Geometry: final body of the model. Coordinates: model frame, mm. Face numbers are marked on the shaded views. A direction names the side the tool comes from. Round coordinates to 2 decimals unless told otherwise and drop trailing zeros. Write each loop counter-clockwise with the first axis right and the second up, starting at its lowest first coordinate (ties: lowest second). Pieces come first, ordered by that corner, then holes. Notation, with made-up numbers: (48, -13) -> (77, -13) arc R15 ccw to (77, 9) -> close; hole circle Ø9 at (53, -15). An arc over 180 degrees is marked (long way). Use one line per item in the form item = value. Start each with the question number.
1. Pin query (flat end, axial travel): pin 1 Ø6 at (y, z) = (8, 1) entering from +X; pin 2 Ø2 at (x, z) = (10, -4) entering from +Y; pin 3 Ø1.6 at (x, y) = (-12, -111.5) entering from +Z. Return the tip coordinate at first contact, or that it passes through.
2. Cut plane B-B, the plane z = -2. Return the cut outline in (x, y).
3. Draft query along Y for the marked faces 3, 4 and 5. Return one class per face: pulls with the +Y half, pulls with the -Y half, needs draft (parallel to the pull), parting line crosses it, or undercut.
4. Cut plane C-C, the plane y = 5. Return the cut outline in (x, z), plus the area to 3 significant figures.
5. Line query: L1, parallel to X at y = -138.5, z = 2.75; L2, parallel to X at y = -138.5, z = 3.75; L3, parallel to Y at x = 7.5, z = -0.75. Output: solid intervals per line, ascending.
6. Reachability of the marked faces 1 and 2 from +Z, -Z, +X, -X, +Y, -Y: full face, straight path, thin tool, end or side. Return the list, or none.
```python
from build123d import *

# Parameters (mm, degrees)
F1_DEPTH = 150
F2_R     = 1.99999
F4_DEPTH = 12.2
F5_DEPTH = 25


# Not quite as in the source:
# - a fillet or chamfer is up to 0.001 mm smaller than in the source, because OpenCascade refuses the exact size


with BuildPart() as f1:
    # F0 (on Front) → F1 (new body)
    with BuildSketch(Plane.XZ):
        with BuildLine():
            ThreePointArc((20, 4.1), (19.4142135624, 5.5142135624), (18, 6.1))
            Line((18, 6.1), (16.25, 6.1))
            ThreePointArc((16.25, 6.1), (15.5428932188, 5.8071067812), (15.25, 5.1))
            Line((15.25, 5.1), (15.25, 3.1))
            Line((15.25, 3.1), (9.25, 3.1))
            Line((9.25, 3.1), (9.25, 5.1))
            ThreePointArc((9.25, 5.1), (8.9571067812, 5.8071067812), (8.25, 6.1))
            Line((8.25, 6.1), (-8.25, 6.1))
            ThreePointArc((-8.25, 6.1), (-8.9571067812, 5.8071067812), (-9.25, 5.1))
            Line((-9.25, 5.1), (-9.25, 3.1))
            Line((-9.25, 3.1), (-15.25, 3.1))
            Line((-15.25, 3.1), (-15.25, 5.1))
            ThreePointArc((-15.25, 5.1), (-15.5428932188, 5.8071067812), (-16.25, 6.1))
            Line((-16.25, 6.1), (-18, 6.1))
            ThreePointArc((-18, 6.1), (-19.4142135624, 5.5142135624), (-20, 4.1))
            Line((-20, 4.1), (-20, -4.1))
            ThreePointArc((-20, -4.1), (-19.4142135624, -5.5142135624), (-18, -6.1))
            Line((-18, -6.1), (18, -6.1))
            ThreePointArc((18, -6.1), (19.4142135624, -5.5142135624), (20, -4.1))
            Line((20, -4.1), (20, 4.1))
        make_face()
    extrude(amount=F1_DEPTH)

    # F2 (radius 2 in the source; OpenCascade refuses exactly that, so slightly less here)
    f2_edges = [f1.edges().sort_by_distance(p)[0] for p in [
        (15.25, -75, 3.1),
        (9.25, -75, 3.1),
        (-9.25, -75, 3.1),
        (-15.25, -75, 3.1),
    ]]
    fillet(f2_edges, radius=F2_R)

    # F3 (on face) → F4 (join)
    with BuildSketch(Plane(origin=(0, 0, -6.1), x_dir=(1, 0, 0), z_dir=(0, 0, -1))):
        with BuildLine():
            Line((0, 0), (-2.5, 0))
            Line((-2.5, 0), (-2.5, -6.5456439427))
            ThreePointArc((-2.5, -6.5456439427), (-1.2794263668, -6.1379979383), (0, -6))
            Line((0, -6), (0, 0))
        make_face()
        with BuildLine():
            Line((2.5, -6.5456439427), (2.5, 0))
            Line((2.5, 0), (0, 0))
            Line((0, 0), (0, -6))
            ThreePointArc((0, -6), (1.2794263668, -6.1379979383), (2.5, -6.5456439427))
        make_face()
        with BuildLine():
            Line((2.5, -8.2583426132), (2.5, -6.5456439427))
            ThreePointArc((2.5, -6.5456439427), (1.2794263668, -6.1379979383), (0, -6))
            Line((0, -6), (0, -7.5))
            ThreePointArc((0, -7.5), (1.3062430401, -7.6937569599), (2.5, -8.2583426132))
        make_face()
        with BuildLine():
            ThreePointArc((0, -6), (-1.2794263668, -6.1379979383), (-2.5, -6.5456439427))
            Line((-2.5, -6.5456439427), (-2.5, -8.2583426132))
            ThreePointArc((-2.5, -8.2583426132), (-1.3062430401, -7.6937569599), (0, -7.5))
            Line((0, -7.5), (0, -6))
        make_face()
        with BuildLine():
            Line((2.5, -15.7416573868), (2.5, -8.2583426132))
            ThreePointArc((2.5, -8.2583426132), (1.3062430401, -7.6937569599), (0, -7.5))
            ThreePointArc((0, -7.5), (-1.3062430401, -7.6937569599), (-2.5, -8.2583426132))
            Line((-2.5, -8.2583426132), (-2.5, -15.7416573868))
            ThreePointArc((-2.5, -15.7416573868), (0, -16.5), (2.5, -15.7416573868))
        make_face()
        with BuildLine():
            ThreePointArc((6, -12), (5.5549205986, -9.7322131619), (4.2857142857, -7.8008747267))
            ThreePointArc((4.2857142857, -7.8008747267), (3.2251093408, -7.7900511001), (3.2142857143, -8.850656045))
            ThreePointArc((3.2142857143, -8.850656045), (4.166190449, -10.2991598715), (4.5, -12))
            ThreePointArc((4.5, -12), (3.9686269666, -14.1213203436), (2.5, -15.7416573868))
            ThreePointArc((2.5, -15.7416573868), (0, -16.5), (-2.5, -15.7416573868))
            ThreePointArc((-2.5, -15.7416573868), (-4.4760183399, -12.4639610121), (-3.2142857143, -8.850656045))
            ThreePointArc((-3.2142857143, -8.850656045), (-3.2251093408, -7.7900511001), (-4.2857142857, -7.8008747267))
            ThreePointArc((-4.2857142857, -7.8008747267), (-2.2677868381, -17.5549205986), (6, -12))
        make_face()
    extrude(amount=-F4_DEPTH)

    # F3 (on face) → F5 (cut)
    with BuildSketch(Plane(origin=(0, 0, -6.1), x_dir=(1, 0, 0), z_dir=(0, 0, -1))):
        with BuildLine():
            ThreePointArc((-4, 143.3023431781), (0, 144.75), (4, 143.3023431781))
            Line((4, 143.3023431781), (4, 150))
            Line((4, 150), (-4, 150))
            Line((-4, 150), (-4, 143.3023431781))
        make_face()
        with BuildLine():
            ThreePointArc((-4, 143.3023431781), (-2.6516504294, 132.8403842887), (6.25, 138.5))
            ThreePointArc((6.25, 138.5), (5.6596157113, 141.1516504294), (4, 143.3023431781))
            ThreePointArc((4, 143.3023431781), (0, 144.75), (-4, 143.3023431781))
        make_face()
    extrude(amount=-F5_DEPTH, mode=Mode.SUBTRACT)


solid = f1.part
```
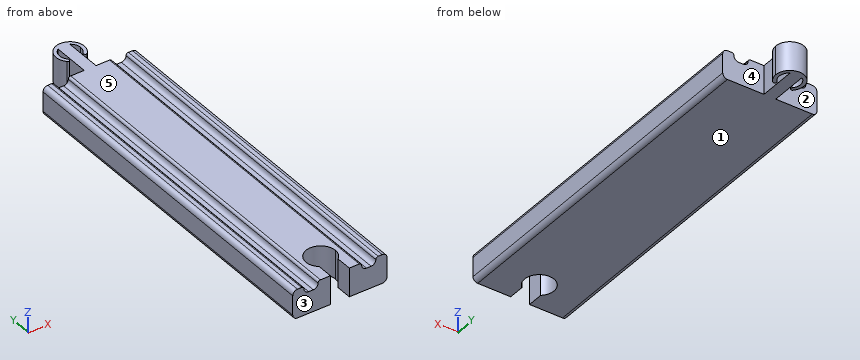
Outcome:
q1.pin_1 = 5.92
q1.pin_2 = 0
q1.pin_3 = 3.1
q2.outline = (-20, -150) -> (-4, -150) -> (-4, -143.3) arc R6.25 cw (long way) to (4, -143.3) -> (4, -150) -> (20, -150) -> (20, 0) -> (2.5, 0) -> (2.5, 15.74) arc R4.5 cw to (3.21, 8.85) arc R0.75 ccw to (4.29, 7.8) arc R6 ccw (long way) to (-4.29, 7.8) arc R0.75 ccw to (-3.21, 8.85) arc R4.5 cw to (-2.5, 15.74) -> (-2.5, 0) -> (-20, 0) -> close
q3.face_3 = pulls with the -Y half
q3.face_4 = undercut
q3.face_5 = needs draft
q4.outline = (-2.5, -6.1) -> (2.5, -6.1) -> (2.5, 6.1) -> (-2.5, 6.1) -> close
q4.area = 61.0 mm^2
q5.L1 = -20 to -6.25, 6.25 to 20
q5.L2 = -20 to -14.73, -9.77 to -6.25, 6.25 to 9.77, 14.73 to 20
q5.L3 = -150 to 0
q6.face_1 = -Z, +X, -X, +Y, -Y
q6.face_2 = +Z, -Z, -X
